Here's the drawing with two shaded views (mm, measured from the low corner). I have some questions. A direction names the side the tool comes from. Give positions to 0.01 mm unless a question says otherwise; leave off trailing zeros. Write each loop counter-clockwise with the first axis right and the second up, starting at its lowest first coordinate (ties: lowest second). Pieces come first, ordered by that corner, then holes.
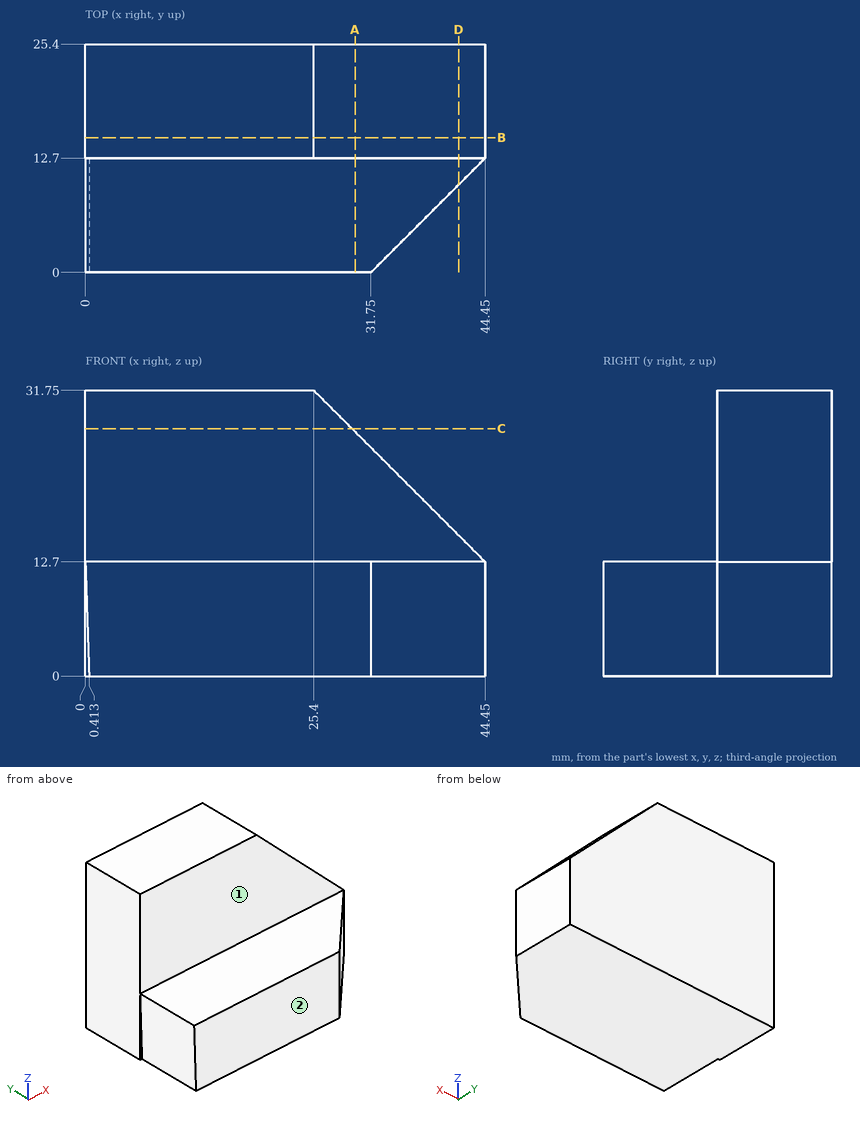
1) For the marked faces 1 and 2, which set-ups out of +Z, -Z, +X, -X, +Y, -Y let a thin tool reach every point of the face, with its end or its side?
Values follow:
face 1: +Z, +X, -X, -Y
face 2: +Z, -Z, +X, -X, -Y
2) Suppose I cut it at A-A on x = 30. Write out the boundary of the cut face in (y, z), plus the area to 3 significant figures.
Values follow:
outline: (0, 0) - (25.4, 0) - (25.4, 27.15) - (12.7, 27.15) - (12.7, 12.7) - (0, 12.7) - close
area: 506 mm2
3) For pin 1 Ø3 at (x, z) = (35, 11.5) entering from -Y; pin 2 Ø1 at (y, z) = (20.5, 24.5) entering from +X; pin 3 Ø6 at (y, z) = (15.5, 26.5) entering from +X; pin 4 Ø12 at (y, z) = (18, 16.5) entering from +X, each with a flat end and sliding along its axis, tell me the tip position at first contact or that it passes through.
Values follow:
pin 1: stops at y = 1.75
pin 2: stops at x = 33.15
pin 3: stops at x = 33.65
pin 4: stops at x = 44.45
4) Please list where these lines run through material, in increasing order: L1, parallel to Z at x = 11.5, y = 5.5; L2, parallel to Y at x = 23, z = 28; L3, parallel to Y at x = 39, z = 3.5.
Values follow:
L1: z = 0 to 12.7
L2: y = 12.7 to 25.4
L3: y = 7.25 to 25.4
5) Suppose I cut it at C-C on z = 27.5. Write out the boundary of the cut face in (x, y).
Values follow:
outline: (0, 12.7) - (29.65, 12.7) - (29.65, 25.4) - (0, 25.4) - close
6) Suppose I cut it at B-B on y = 15. Write out the boundary of the cut face in (x, z), plus the area to 3 significant figures.
Values follow:
outline: (0, 0) - (44.45, 0) - (44.45, 12.7) - (25.4, 31.75) - (0, 31.75) - close
area: 1,230 mm2
7) Suppose I cut it at D-D on x = 41.5. Write out the boundary of the cut face in (y, z).
Values follow:
outline: (9.75, 0) - (25.4, 0) - (25.4, 15.65) - (12.7, 15.65) - (12.7, 12.7) - (9.75, 12.7) - close
